Can you work these out from the model? Positions are in its coordinate system, mm. A direction names the side the tool comes from. Give positions to 0.01 mm unless a question says otherwise; leave off trailing zeros. Order: outer loops, then holes, each group sorted by start corner. A loop starts at its lowest first (then second) coordinate and runs counter-clockwise, first axis right, second up.
```python
from build123d import *

# Parameters (mm, degrees)
SKETCH1_R               = 36.96335
BOSS_EXTRUDE1_DEPTH     = 171.45
FILLET1_R               = 2.54
SKETCH10_R              = 36.96335
BOSS_EXTRUDE2_DEPTH     = 25.4
FILLET2_R               = 19.05
SKETCH11_R              = 21.36775
BOSS_EXTRUDE3_DEPTH     = 25.4
FILLET3_R               = 2.54
SKETCH12_R              = 17.78
CUT_EXTRUDE1_DEPTH      = 221.742
SKETCH13_R              = 35.56
CUT_EXTRUDE2_DEPTH      = 171.45
CUT_EXTRUDE3_DEPTH      = 229.314784975
CUT_EXTRUDE3_DEPTH_BACK = 2.54
SKETCH15_R              = 7.62


with BuildPart() as part:
    # Sketch1 → Boss-Extrude1 (new body)
    with BuildSketch(Plane(origin=(0, 0, 0), x_dir=(1, 0, 0), z_dir=(0, 1, 0))):
        with Locations(Location((0, 0, 0), (0, 0, 270))):
            Circle(SKETCH1_R)
    extrude(amount=BOSS_EXTRUDE1_DEPTH)

    # Fillet1
    fillet1_edges = [part.edges().sort_by_distance(p)[0] for p in [
        (0, 0, -36.96335),
    ]]
    fillet(fillet1_edges, radius=FILLET1_R)

    # Sketch10 → Boss-Extrude2 (add)
    with BuildSketch(Plane(origin=(0, 171.45, 0), x_dir=(1, 0, 0), z_dir=(0, 1, 0))):
        with Locations(Location((0, 0, 0), (0, 0, 270))):
            Circle(SKETCH10_R)
    extrude(amount=BOSS_EXTRUDE2_DEPTH)

    # Fillet2
    fillet2_edges = [part.edges().sort_by_distance(p)[0] for p in [
        (0, 196.85, -36.96335),
    ]]
    fillet(fillet2_edges, radius=FILLET2_R)

    # Sketch11 → Boss-Extrude3 (add)
    with BuildSketch(Plane(origin=(0, 196.85, 0), x_dir=(1, 0, 0), z_dir=(0, 1, 0))):
        with Locations(Location((0, 0, 0), (0, 0, 270))):
            Circle(SKETCH11_R)
    extrude(amount=BOSS_EXTRUDE3_DEPTH)

    # Fillet3
    fillet3_edges = [part.edges().sort_by_distance(p)[0] for p in [
        (0, 222.25, -21.36775),
    ]]
    fillet(fillet3_edges, radius=FILLET3_R)

    # Sketch12 → Cut-Extrude1 (cut)
    with BuildSketch(Plane(origin=(0, 222.25, 0), x_dir=(1, 0, 0), z_dir=(0, 1, 0))):
        with Locations(Location((0, 0, 0), (0, 0, 270))):
            Circle(SKETCH12_R)
    extrude(amount=-CUT_EXTRUDE1_DEPTH, mode=Mode.SUBTRACT)

    # Sketch13 → Cut-Extrude2 (cut)
    with BuildSketch(Plane(origin=(0, 0.508, 0), x_dir=(1, 0, 0), z_dir=(0, 1, 0))):
        with Locations(Location((0, 0, 0), (0, 0, 270))):
            Circle(SKETCH13_R)
    extrude(amount=CUT_EXTRUDE2_DEPTH, mode=Mode.SUBTRACT)

    # Sketch14 → Cut-Revolve1 (revolve, cut)
    with BuildSketch(Plane.XY, mode=Mode.PRIVATE) as cut_revolve1_sk:
        with BuildLine():
            Line((35.56, 171.958), (0, 171.958))
            Line((0, 171.958), (0, 196.85))
            Line((0, 196.85), (16.51, 196.85))
            ThreePointArc((16.51, 196.85), (29.980384182, 191.270384182), (35.56, 177.8))
            Line((35.56, 177.8), (35.56, 171.958))
        make_face()
    revolve(cut_revolve1_sk.sketch.rotate(Axis((0, 171.958, 0), (0, 1, 0)), 90), axis=Axis((0, 171.958, 0), (0, 1, 0)), mode=Mode.SUBTRACT)

    # Sketch15 → Cut-Extrude3 (cut, two sides: drawn at the far end of the back side and taken through both)
    with BuildSketch(Plane(origin=(0, 0, 0), x_dir=(0, 0, -1), z_dir=(1, 0, 0)).offset(-CUT_EXTRUDE3_DEPTH_BACK)):
        with Locations(Location((0, 139.7, 0), (0, 0, 180))):
            Circle(SKETCH15_R)
    extrude(amount=CUT_EXTRUDE3_DEPTH + CUT_EXTRUDE3_DEPTH_BACK, mode=Mode.SUBTRACT)


solid = part.part
```
1) We'd pull the mould along Y, two halves only. Please class faces 4 (the face through (-8.18, 208.12, 19.74)), 5 (the face through (36, 135, -6)), 6 (the face through (0, 0, 0)): +Y half, -Y half, draft (parallel to the pull), parting line (faces both ways), or undercut.
2) Which directions (+Z, -Z, +X, -X, +Y, -Y) give clear straight access to the entire face, cutting with the end or side of a thin tool? Please do faces 1 (the face through (0, 0.508, 0)), 2 (the face through (-17.36, 209.71, -3.85)), 3 (the face through (1.625, 88.943, -36.928)).
3) Suppose I cut it at A-A (y = 57.5). Please give me the cut outline in (x, z).
4) I'm going to push flat-ended pins straight in: pin 1 Ø9 at (y, z) = (139.7, 0) entering from -X; pin 2 Ø8 at (x, z) = (23.5, 16.5) entering from +Y; pin 3 Ø5 at (y, z) = (119, 25.5) entering from -X. Where does each tip first touch, or does it pass through?
5) Suppose I cut it at B-B (y = 204). Please give me the cut outline in (x, z), and give its area (3 significant figures).
6) Suppose I cut it at C-C (y = 139.7). Please give me the cut outline in (x, z), and give its area (3 significant figures).
7) If I drill on line 1 (X direction, y = 153, z = 0.5); line 2 (X direction, y = 215, z = 0); line 3 (Y direction, x = 9.5, z = 10.5), over which ranges is the centre line in solid material (lowest first)?
Results:
1. face 4: draft
1. face 5: undercut
1. face 6: -Y half
2. face 1: none
2. face 2: +Y
2. face 3: +Y, -Y
3. outline: circle Ø73.93 at (0, 0); hole circle Ø71.12 at (0, 0)
4. pin 1: stops at x = -36.96
4. pin 2: stops at y = 195.59
4. pin 3: stops at x = -28.94
5. outline: circle Ø42.74 at (0, 0); hole circle Ø35.56 at (0, 0)
5. area: 441 mm2
6. outline: (34.73, -7.62) arc R35.56 cw (long way) to (34.73, 7.62) - (36.17, 7.62) arc R36.96 ccw (long way) to (36.17, -7.62) - close
6. area: 298 mm2
7. line 1: x = -36.96 to -35.56, 35.56 to 36.96
7. line 2: x = -21.37 to -17.78, 17.78 to 21.37
7. line 3: y = 0 to 0.51
